```python
from build123d import *

# Parameters (mm, degrees)
SKETCH1_R           = 3.3
SKETCH1_W           = 2
SKETCH1_H           = 14
BOSS_EXTRUDE1_DEPTH = 2


with BuildPart() as part:
    # Sketch1 → Boss-Extrude1 (new body)
    with BuildSketch(Plane.XY):
        with BuildLine():
            Line((-19.253359056, 9.714066104), (-19.253359056, -6.489091482))
            ThreePointArc((-19.253359056, -6.489091482), (-11.269151238, -12.206183048), (-2.097048594, -15.714066104))
            Line((-2.097048594, -15.714066104), (-2.097048594, 13.714066104))
            Line((-2.097048594, 13.714066104), (-11.075689526, 13.714066104))
            Line((-11.075689526, 13.714066104), (-11.075689526, 15.714066104))
            Line((-11.075689526, 15.714066104), (-31.04567167, 15.714066104))
            ThreePointArc((-31.04567167, 15.714066104), (-27.656648188, 4.883682523), (-21.253359056, -4.485446411))
            Line((-21.253359056, -4.485446411), (-21.253359056, 9.714066104))
            Line((-21.253359056, 9.714066104), (-19.253359056, 9.714066104))
        make_face()
        with Locations((-10.753359056, 4.036396574)):
            Circle(SKETCH1_R, mode=Mode.SUBTRACT)
        with Locations((-4.097048594, 2.714066104)):
            Rectangle(SKETCH1_W, SKETCH1_H, mode=Mode.SUBTRACT)
    extrude(amount=BOSS_EXTRUDE1_DEPTH)


solid = part.part
```
Can you work these out from the model? Positions are in its coordinate system, mm. A direction names the side the tool comes from. Coordinates: 2 decimals unless noted, no trailing zeros. Order: outer loops, then holes, each group sorted by start corner. A loop starts at its lowest first (then second) coordinate and runs counter-clockwise, first axis right, second up. Notation, with made-up numbers: (8.25, 12.5) -> (64.25, 12.5) arc R18 cw to (64.25, 28.5) -> close; hole circle Ø9 at (81.5, 5). An arc over 180 degrees is marked (long way). Write each question's results on one line, items separated by ' | '.
Item 1: I'm going to push flat-ended pins straight in: pin 1 Ø1 at (x, z) = (-20, 1.5) entering from -Y; pin 2 Ø1 at (x, z) = (-28, 1.5) entering from -Y; pin 3 Ø1 at (x, y) = (-6.5, 10.5) entering from -Z; pin 4 Ø1 at (x, z) = (-4.5, 1) entering from -Y. Where does each tip first touch, or does it pass through?
Results are:
pin 1: y = 9.71 | pin 2: y = 4.56 | pin 3: z = 0 | pin 4: y = -15.2
Item 2: If we mould it in two halves opening along X, with no side actions, what happens to faces 1 (the face through (-17, 4, 2)), 2 (the face through (-27.726, 5.027, 0.986)), 3 (the face through (-4, 9.714, 1)), 4 (the face through (-11.076, 15, 1))? For each: +X half, -X half, draft (parallel to the pull), parting line (faces both ways), or undercut.
Results are:
face 1: draft | face 2: -X half | face 3: undercut | face 4: +X half
Item 3: If I drill on line 1 along X through (y, z) = (9, 0.2); line 2 along X through (y, z) = (2, 0.25); line 3 along X through (y, z) = (1, 1.6), over which ranges is the centre line in solid material (lowest first)?
Results are:
line 1: -29.37 to -21.25, -19.25 to -5.1, -3.1 to -2.1 | line 2: -26.1 to -21.25, -19.25 to -13.35, -8.16 to -5.1, -3.1 to -2.1 | line 3: -25.49 to -21.25, -19.25 to -12.05, -9.46 to -5.1, -3.1 to -2.1
Item 4: I want a section at B-B, the plane z = 0.85. Write out the boundary of the cut face in (x, y), then the cut area to 3 significant figures.
Results are:
outline: (-31.05, 15.71) arc R38.45 ccw to (-21.25, -4.49) -> (-21.25, 9.71) -> (-19.25, 9.71) -> (-19.25, -6.49) arc R38.45 ccw to (-2.1, -15.71) -> (-2.1, 13.71) -> (-11.08, 13.71) -> (-11.08, 15.71) -> close; hole circle Ø6.6 at (-10.75, 4.04); hole (-5.1, -4.29) -> (-3.1, -4.29) -> (-3.1, 9.71) -> (-5.1, 9.71) -> close | area: 532 mm²
Item 5: I want a section at A-A, the plane y = -3.5. Write out the boundary of the cut face in (x, z), then the cut area to 3 significant figures.
Results are:
outline: (-22.14, 0) -> (-21.25, 0) -> (-21.25, 2) -> (-22.14, 2) -> close; (-19.25, 0) -> (-5.1, 0) -> (-5.1, 2) -> (-19.25, 2) -> close; (-3.1, 0) -> (-2.1, 0) -> (-2.1, 2) -> (-3.1, 2) -> close | area: 32.1 mm²
Item 6: I want a section at C-C, the plane x = -8.25. Write out the boundary of the cut face in (y, z), then the cut area to 3 significant figures.
Results are:
outline: (-13.66, 0) -> (1.89, 0) -> (1.89, 2) -> (-13.66, 2) -> close; (6.19, 0) -> (13.71, 0) -> (13.71, 2) -> (6.19, 2) -> close | area: 46.2 mm²
Item 7: I want a section at D-D, the plane y = 9. Write out the boundary of the cut face in (x, z).
Results are:
outline: (-29.37, 0) -> (-21.25, 0) -> (-21.25, 2) -> (-29.37, 2) -> close; (-19.25, 0) -> (-5.1, 0) -> (-5.1, 2) -> (-19.25, 2) -> close; (-3.1, 0) -> (-2.1, 0) -> (-2.1, 2) -> (-3.1, 2) -> close
Item 8: Which directions (+Z, -Z, +X, -X, +Y, -Y) give clear straight access to the entire face, cutting with the end or side of a thin tool? Please do faces 5 (the face through (-21, 15.714, 1)), 6 (the face through (-7, 13.714, 1)), 7 (the face through (-4, -4.286, 1)), 8 (the face through (-11.39, -12.14, 0.99)), 9 (the face through (-20, 9.714, 1)).
Results are:
face 5: +Z, -Z, +X, -X, +Y | face 6: +Z, -Z, +X, +Y | face 7: +Z, -Z | face 8: +Z, -Z, -X, -Y | face 9: +Z, -Z, -Y
